Geometry check sheet. Reference: the model listing, model coordinates, mm. A direction names the side the tool comes from. Coordinates: 2 decimals unless noted, no trailing zeros. Loops run counter-clockwise (first coordinate to the right, second up) from the corner with the lowest first, then second, coordinate; pieces in that order, holes last. Notation, with made-up numbers: (69, 46.25) - (104, 46.25) arc R16 cw to (104, 50.25) - close; hole circle Ø10 at (-15, 7.5). An arc over 180 degrees is marked (long way). Write each question's results on one line, items separated by ' | '. Start each with the question number.
(1) Material ranges on probe 1 along X at (y, z) = (2.5, -7.75); probe 2 along Z at (x, y) = (8.5, 11.5); probe 3 along Z at (x, y) = (8, 2.75), recorded low to high.
(2) Sectioned sample at A-A (y = 4.5). Enter the section's corners in (x, z), plus the area to 3 significant figures.
(3) Sectioned sample at B-B (z = -8). Enter the section's corners in (x, y).
(4) Access from +Z, -Z, +X, -X, +Y, -Y to the whole of each face (thin tool, end or side, straight path). Record for faces 1 (the face through (13, 6, -1.129)), 2 (the face through (16, 9, -3)), 3 (the face through (7.625, 5.916, -1.352)), 4 (the face through (-16, 4, -3)), 5 (the face through (-13, 5, -3)).
(5) Go/stop test with flat-tipped pins: pin 1 Ø2.5 at (x, y) = (-13.5, 6) entering from +Z; pin 2 Ø0.9 at (x, z) = (16.5, -2.5) entering from -Y; pin 3 Ø2.5 at (x, z) = (-1.43, -7.63) entering from +Y; pin 4 Ø0.9 at (x, z) = (-12.5, -2) entering from +Y. Record where each tip stops, or that it passes through.
(6) Mould release check, pull along Z, two halves, no side actions. Record for faces 6 (the face through (8.246, 6.409, -9.093)), 7 (the face through (4.5, 12, -5.4)), 8 (the face through (-13, 6, -1.129)), 9 (the face through (-17.429, 7, -3)): pulls with the +Z half, pulls with the -Z half, needs draft (parallel to the pull), parting line crosses it, or undercut.
(7) Sectioned sample at D-D (x = 2). Enter the section's corners in (y, z), plus the area to 3 significant figures.
(8) Sectioned sample at C-C (x = 9.5). Enter the section's corners in (y, z), plus the area to 3 significant figures.
Autodesk Inventor part; units mm, degrees
ref_plane "YZ Plane" through (0, 0, 0) normal (1, 0, 0) x (0, 1, 0)
ref_plane "XZ Plane" through (0, 0, 0) normal (0, 1, 0) x (-1, 0, 0)
ref_plane "XY Plane" through (0, 0, 0) normal (0, 0, 1) x (1, 0, 0)
sketch "Esquisse1" plane through (0, 0, 0) normal (0, 1, 0) x (-1, 0, 0)
  line L0 (4.4286, 5.3714) -> (-11.5714, 5.3714)
  line L1 (-11.5714, 5.3714) -> (-11.5714, -10.6286)
  line L2 (-11.5714, -10.6286) -> (4.4286, -10.6286)
  line L3 (4.4286, -10.6286) -> (4.4286, 5.3714)
  point P0 (0, 0)
  dimension "d0" = 16
  dimension "d1" = 16
extrude "Extrusion1" add sketch "Esquisse1" along normal blind 13
sketch "Esquisse2" plane through (0, 0, 0) normal (0, -1, 0) x (1, 0, 0)
  circle A0 centre (3.5714, -2.6286) radius 4.25
  line L0 (-4.4286, 5.3714) -> (11.5714, 5.3714)
  line L1 (11.5714, 5.3714) -> (11.5714, -10.6286)
  point P0 (0, 0)
  dimension "d4" = 8
  dimension "d5" = 8
  dimension "d6" = 8.5
extrude "Extrusion2" cut sketch "Esquisse2" against normal blind 12
sketch "Esquisse3" plane through (3.5714, 12, -2.6286) normal (0, -1, 0) x (1, 0, 0)
  circle A0 centre (0, 0) radius 2.75
  line L0 (8, -8) -> (-8, -8)
  line L1 (8, 8) -> (8, -8)
  point P0 (-3.5714, 2.6286)
  dimension "d9" = 5.5
  dimension "d10" = 8
  dimension "d11" = 8
extrude "Extrusion3" cut sketch "Esquisse3" against normal through all
sketch "Esquisse4" plane through (0, 0, 0) normal (0, -1, 0) x (1, 0, 0)
  circle A0 centre (8.5714, 2.3714) radius 1.5
  circle A1 centre (-1.4286, 2.3714) radius 1.5
  circle A2 centre (-1.4286, -7.6286) radius 1.5
  circle A3 centre (8.5714, -7.6286) radius 1.5
  line L0 (-4.4286, -10.6286) -> (-4.4286, 5.3714)
  line L1 (-4.4286, 5.3714) -> (11.5714, 5.3714)
  line L2 (11.5714, 5.3714) -> (11.5714, -10.6286)
  line L3 (11.5714, -10.6286) -> (-4.4286, -10.6286)
  point P0 (0, 0)
  dimension "d14" = 3
  dimension "d15" = 3
  dimension "d16" = 3
  dimension "d17" = 3
  dimension "d19" = 3
  dimension "d20" = 3
  dimension "d21" = 3
  dimension "d22" = 3
  dimension "d23" = 3
  dimension "d24" = 3
  dimension "d25" = 3
  dimension "d26" = 3
extrude "Extrusion4" cut sketch "Esquisse4" against normal through all contours A0 | A1 | A2 | A3
sketch "Esquisse6" plane through (11.5714, 0, 5.3714) normal (1, 0, 0) x (0, 0, -1)
  line L0 (6.5, 8) -> (9.5, 8)
  line L1 (9.5, 8) -> (9.5, 5)
  line L2 (9.5, 5) -> (6.5, 5)
  line L3 (6.5, 5) -> (6.5, 8)
  line L4 (0, 0) -> (0, 13)
  line L5 (0, 13) -> (16, 13)
  point P0 (5.3714, 0)
  dimension "d29" = 3
  dimension "d30" = 3
  dimension "d31" = 6.5
  dimension "d32" = 5
extrude "Extrusion5" add sketch "Esquisse6" along normal blind 3
sketch "Esquisse7" plane through (14.5714, 0, 5.3714) normal (1, 0, 0) x (0, 0, -1)
  line L0 (5.5, 9) -> (10.5, 9)
  line L1 (10.5, 9) -> (10.5, 4)
  line L2 (10.5, 4) -> (5.5, 4)
  line L3 (5.5, 4) -> (5.5, 9)
  line L4 (0, 13) -> (16, 13)
  line L5 (0, 0) -> (0, 13)
  point P0 (5.3714, 0)
  dimension "d35" = 5
  dimension "d36" = 5
  dimension "d37" = 4
  dimension "d38" = 5.5
extrude "Extrusion6" add sketch "Esquisse7" along normal blind 3
sketch "Esquisse8" plane through (-4.4286, 0, -10.6286) normal (-1, 0, 0) x (0, 0, 1)
  line L0 (0, 0) -> (0, 13)
  line L1 (0, 13) -> (16, 13)
  line L2 (16, 13) -> (16, 0)
  line L3 (16, 0) -> (0, 0)
  line L4 (0, 0) -> (0, 13)
  point P0 (10.6286, 0)
extrude "Extrusion7" add sketch "Esquisse8" along normal blind 7
sketch "Esquisse9" plane through (-11.4286, 0, -10.6286) normal (-1, 0, 0) x (0, 0, 1)
  line L0 (9.5, 8) -> (6.5, 8)
  line L1 (6.5, 8) -> (6.5, 5)
  line L2 (6.5, 5) -> (9.5, 5)
  line L3 (9.5, 5) -> (9.5, 8)
  line L4 (16, 0) -> (16, 13)
  line L5 (16, 13) -> (0, 13)
  point P0 (10.6286, 0)
  dimension "d43" = 6.5
  dimension "d44" = 5
  dimension "d45" = 3
  dimension "d46" = 3
extrude "Extrusion8" add sketch "Esquisse9" along normal blind 3
sketch "Esquisse10" plane through (-14.4286, 0, -10.6286) normal (-1, 0, 0) x (0, 0, 1)
  line L0 (10.5, 9) -> (5.5, 9)
  line L1 (5.5, 9) -> (5.5, 4)
  line L2 (5.5, 4) -> (10.5, 4)
  line L3 (10.5, 4) -> (10.5, 9)
  line L4 (16, 0) -> (16, 13)
  line L5 (0, 0) -> (16, 0)
  point P0 (10.6286, 0)
  dimension "d49" = 5.5
  dimension "d50" = 4
  dimension "d51" = 5
  dimension "d52" = 5
extrude "Extrusion9" add sketch "Esquisse10" along normal blind 3
properties part number "capuchon_roulement"
Outcome:
1) probe 1: x = -11.43 to -2.92, 0.07 to 7.08, 10.07 to 11.57 | probe 2: z = -10.63 to -9.13, -6.13 to 0.87, 3.87 to 5.37 | probe 3: z = -10.63 to -9.02, -6.24 to 0.98, 3.76 to 5.37
2) outline: (-17.43, -5.13) - (-14.43, -5.13) - (-14.43, -0.13) - (-17.43, -0.13) - close; (-11.43, -10.63) - (11.57, -10.63) - (11.57, 5.37) - (-11.43, 5.37) - close; (14.57, -5.13) - (17.57, -5.13) - (17.57, -0.13) - (14.57, -0.13) - close; hole circle Ø3 at (-1.43, -7.63); hole circle Ø3 at (-1.43, 2.37); hole circle Ø8.5 at (3.57, -2.63); hole circle Ø3 at (8.57, -7.63); hole circle Ø3 at (8.57, 2.37) | area: 313 mm2
3) outline: (-11.43, 0) - (-2.88, 0) - (-2.88, 13) - (-11.43, 13) - close; (0.02, 0) - (7.12, 0) - (7.12, 13) - (0.02, 13) - close; (10.02, 0) - (11.57, 0) - (11.57, 13) - (10.02, 13) - close
4) face 1: +Z, +Y, -Y | face 2: +Z, -Z, +X, +Y | face 3: -Y | face 4: +Z, -Z, -X, -Y | face 5: +Z, -Z, -Y
5) pin 1: stops at z = -0.13 | pin 2: stops at y = 4 | pin 3: passes through | pin 4: stops at y = 8
6) face 6: undercut | face 7: undercut | face 8: pulls with the +Z half | face 9: needs draft
7) outline: (0, -10.63) - (13, -10.63) - (13, -4.89) - (12, -4.89) - (12, -6.58) - (0, -6.58) - close; (0, 1.32) - (12, 1.32) - (12, -0.37) - (13, -0.37) - (13, 5.37) - (0, 5.37) - close | area: 109 mm2
8) outline: (0, -10.63) - (13, -10.63) - (13, -8.81) - (0, -8.81) - close; (0, -6.45) - (13, -6.45) - (13, 1.19) - (0, 1.19) - close; (0, 3.55) - (13, 3.55) - (13, 5.37) - (0, 5.37) - close | area: 147 mm2
